Design review of the part built by this model. Coordinates are the model's own, in mm. A direction names the side the tool comes from. Give positions to 0.01 mm unless a question says otherwise; leave off trailing zeros. Write each loop counter-clockwise with the first axis right and the second up, starting at its lowest first coordinate (ties: lowest second). Pieces come first, ordered by that corner, then holes. Notation, with made-up numbers: (3.5, 81) -> (51.5, 81) arc R14 ccw to (51.5, 86) -> close; hole circle Ø1 at (73, 61). An arc over 180 degrees is marked (long way). Use CSV: the item, a comma, the result in double quotes.
```python
from build123d import *

# Parameters (mm, degrees)
F0_W     = 83.6216490716
F0_H     = 83.1985995173
F1_DEPTH = 40
F2_W     = 41.8108245358
F2_H     = 83.1985995173
F3_DEPTH = 40
F4_SIZE  = 10


with BuildPart() as f1:
    # F0 (on Top) → F1 (new body)
    with BuildSketch(Plane.XY):
        with Locations((-17.3164242879, -4.335001111)):
            Rectangle(F0_W, F0_H)
    extrude(amount=F1_DEPTH)

    # F2 (on face) → F3 (join)
    with BuildSketch(Plane.XY.offset(40)):
        with Locations((-38.2218365557, -4.335001111)):
            Rectangle(F2_W, F2_H)
    extrude(amount=F3_DEPTH)

    # F4
    f4_edges = [f1.edges().sort_by_distance(p)[0] for p in [
        (-17.316424, -4.335001, 80),
        (-38.221837, -45.934301, 80),
        (-59.127249, -4.335001, 80),
        (-38.221837, 37.264299, 80),
        (-17.316424, -45.934301, 60),
        (-17.316424, -4.335001, 40),
        (-17.316424, 37.264299, 60),
        (3.588988, 37.264299, 40),
        (3.588988, -45.934301, 40),
        (24.4944, -4.335001, 40),
        (24.4944, -45.934301, 20),
        (24.4944, 37.264299, 20),
        (24.4944, -4.335001, 0),
        (-17.316424, -45.934301, 0),
        (-59.127249, -45.934301, 40),
        (-59.127249, -4.335001, 0),
        (-17.316424, 37.264299, 0),
        (-59.127249, 37.264299, 40),
    ]]
    chamfer(f4_edges, length=F4_SIZE)


solid = f1.part
```
(1) Take a section at C-C (x = -40). Write out the cut boundary in (y, z), then the cut area to 3 significant figures.
Established:
outline,"(-45.93, 10) -> (-35.93, 0) -> (27.26, 0) -> (37.26, 10) -> (37.26, 70) -> (27.26, 80) -> (-35.93, 80) -> (-45.93, 70) -> close"
area,"6,460 mm2"
(2) Take a section at B-B (y = 9). Write out the cut boundary in (x, z).
Established:
outline,"(-59.13, 10) -> (-49.13, 0) -> (14.49, 0) -> (24.49, 10) -> (24.49, 30) -> (14.49, 40) -> (-7.32, 40) -> (-17.32, 50) -> (-17.32, 70) -> (-27.32, 80) -> (-49.13, 80) -> (-59.13, 70) -> close"
(3) Take a section at D-D (z = 33.5). Write out the cut boundary in (x, y).
Established:
outline,"(-59.13, -35.93) -> (-49.13, -45.93) -> (-10.82, -45.93) -> (-7.32, -42.43) -> (14.49, -42.43) -> (20.99, -35.93) -> (20.99, 27.26) -> (14.49, 33.76) -> (-7.32, 33.76) -> (-10.82, 37.26) -> (-49.13, 37.26) -> (-59.13, 27.26) -> close"
(4) Take a section at A-A (z = 53). Write out the cut boundary in (x, y), then the cut area to 3 significant figures.
Established:
outline,"(-59.13, -35.93) -> (-49.13, -45.93) -> (-27.32, -45.93) -> (-17.32, -35.93) -> (-17.32, 27.26) -> (-27.32, 37.26) -> (-49.13, 37.26) -> (-59.13, 27.26) -> close"
area,"3,280 mm2"
(5) Clearance check with flat-ended pins moving along their axes: pin 1 (1.5 mm diameter, centred on x = -15.5, z = 45, fed in from -Y); pin 2 (22 mm diameter, centred on y = 1, z = 64.5, fed in from +X); pin 3 (1 mm diameter, centred on x = -50, y = 14, fed in from +Z). State where each tip first meets the part, or that it passes through.
Established:
pin 1,"stops at y = -40.18"
pin 2,"stops at x = -17.32"
pin 3,"stops at z = 79.63"
(6) For line 1 along X through (y, z) = (-6.5, 50); line 2 along Z through (x, y) = (-14, 15.5); line 3 along Y through (x, z) = (-16, 42), list the stretches that pass through material, from the lowest coordinate up. Write a range as [from, to].
Established:
line 1,"x = [-59.13, -17.32]"
line 2,"z = [0, 46.68]"
line 3,"y = [-42.62, 33.95]"
(7) Tool access review of faces 1 (the face through (-22.246, 32.194, 59.86)), 2 (the face through (3.436, -40.864, 35.07)), 3 (the face through (24.494, -5, 20)): name each direction out of +Z, -Z, +X, -X, +Y, -Y from which nothing blocks a thin tool from reaching the whole face with its end or side.
Established:
face 1,"+Z, +X, +Y"
face 2,"+Z, +X, -Y"
face 3,"+Z, -Z, +X, +Y, -Y"
